The model under review builds one solid part; all positions refer to its coordinate system, in mm. Face numbers are marked on the shaded views. Round coordinates to 2 decimals unless told otherwise and drop trailing zeros. Order: outer loops, then holes, each group sorted by start corner. A loop starts at its lowest first (then second) coordinate and runs counter-clockwise, first axis right, second up. Notation, with made-up numbers: (-24, 50.5) - (17, 50.5) arc R13 ccw to (17, 68.5) - close; hole circle Ø11 at (-16.5, -27.75). An arc over 180 degrees is marked (long way). One line per question, with ' | ' between items. Start each with the question number.
Item 1: Insertion check: pin 1 Ø7.5 at (y, z) = (-39.02, 37.58) entering from -X; pin 2 Ø15 at (x, y) = (112.5, -36) entering from +Z; pin 3 Ø1 at (y, z) = (-26.5, 31.5) entering from +X. Each pin has a flat end and moves straight along its axis. Give the tip position at first contact, or say it passes through.
Item 2: For L1, parallel to Z at x = 89.5, y = -28.5; L2, parallel to Y at x = 39, z = 42.5; L3, parallel to Z at x = 17, y = -39, list the stretches that pass through material, from the lowest coordinate up. Write a range as [from, to].
Item 3: Add section A-A on z = 39. State the section outline as (x, y) points (3 decimals), and give its area (3 significant figures).
Item 4: Add section B-B on x = 37. State the section outline as (y, z) points.
Item 5: Add section C-C on y = -6. State the section outline as (x, z) points.
Item 6: Draft analysis for pull direction X (two halves, no side actions). For the marked faces 1, 2, 3 and 4, state which applies: +X half, -X half, draft (parallel to the pull), parting line (faces both ways), or undercut.
Item 7: Add section D-D on x = 51. State the section outline as (y, z) points.
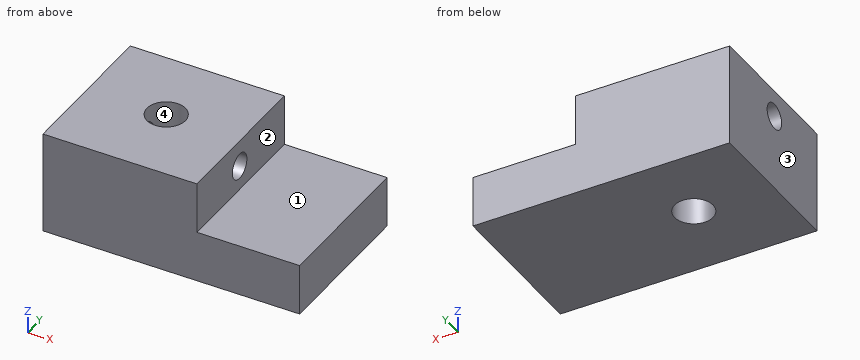
from build123d import *

# Parameters (mm, degrees)
F1_DEPTH = 76.2
F2_DEPTH = 25.4
F4_D     = 19.05
F6_D     = 12.7


with BuildPart() as f1:
    # F0 (on Front) → F1 (new body)
    with BuildSketch(Plane.XZ):
        Polygon((0, 50.8), (0, 0), (127, 0), (127, 25.4), (76.2, 25.4), (76.2, 50.8), align=None)
    extrude(amount=F1_DEPTH)

    # F0 (on Front) → F2 (join)
    with BuildSketch(Plane.XZ):
        Polygon((0, 50.8), (0, 0), (127, 0), (127, 25.4), (76.2, 25.4), (76.2, 50.8), align=None)
    extrude(amount=F2_DEPTH)

    # F4 (through all)
    with Locations(Plane.XY.offset(50.8)):
        with Locations((38.853236, -37.206624)):
            Hole(F4_D / 2)

    # F6 (through all)
    with Locations(Plane.YZ.offset(76.2)):
        with Locations((-39.024234, 37.578892)):
            Hole(F6_D / 2)


solid = f1.part
Determined:
1) pin 1: through | pin 2: z = 25.4 | pin 3: x = 76.2
2) L1: [0, 25.4] | L2: [-76.2, -46.73], [-27.68, 0] | L3: [0, 31.23], [43.93, 50.8]
3) outline: (0, -76.2) - (76.2, -76.2) - (76.2, -45.213) - (44.013, -45.213) arc R9.525 cw to (33.694, -45.213) - (0, -45.213) - close; (0, -32.835) - (30.391, -32.835) arc R9.525 cw to (47.316, -32.835) - (76.2, -32.835) - (76.2, 0) - (0, 0) - close | area: 4,790 mm2
4) outline: (-76.2, 0) - (-46.55, 0) - (-46.55, 50.8) - (-76.2, 50.8) - close; (-27.86, 0) - (0, 0) - (0, 50.8) - (-27.86, 50.8) - close
5) outline: (0, 0) - (127, 0) - (127, 25.4) - (76.2, 25.4) - (76.2, 50.8) - (0, 50.8) - close
6) face 1: draft | face 2: +X half | face 3: -X half | face 4: undercut
7) outline: (-76.2, 0) - (0, 0) - (0, 50.8) - (-76.2, 50.8) - close; hole circle Ø12.7 at (-39.02, 37.58)
